For this review, take the finished solid that the model builds, in its own axes (mm). A direction names the side the tool comes from. Coordinates: 2 decimals unless noted, no trailing zeros. Loops run counter-clockwise (first coordinate to the right, second up) from the corner with the lowest first, then second, coordinate; pieces in that order, holes last. Notation, with made-up numbers: (24, -13.75) - (81, -13.75) arc R19 ccw to (81, 13.25) - close; hole circle Ø3 at (16.5, 10.5). An arc over 180 degrees is marked (long way). One line per item, written item: value. Start each with the question number.
1. The part is to be moulded in two halves that separate along Y. For faces 3 (the face through (-1.46, 7.41, -35.94)), 4 (the face through (-1.46, 69.41, -35.94)), 5 (the face through (0, 0, -36)), 6 (the face through (-50, 197, -20)), say which applies: released by +Y, released by -Y, zero draft, split by the parting line, or undercut.
2. Insertion check: pin 1 (17.5 mm diameter, centred on x = 0, y = 14, fed in from -Z); pin 2 (23.5 mm diameter, centred on x = 9.5, y = 253.5, fed in from +Z). Each pin has a flat end and moves straight along its axis. Give the tip position at first contact, or say it passes through.
3. Take a section at D-D, the plane y = 366. State the section outline as (x, z) points, and give its area (3 significant figures).
4. Take a section at A-A, the plane z = -16. State the section outline as (x, y) points.
5. For faces 1 (the face through (42, 197, -15)), 2 (the face through (3.63, 391.69, -35.94)), list the 3-axis set-ups (+Z, -Z, +X, -X, +Y, -Y) from which the entire face can be reached by the end or side of a thin tool; tool diameter is ignored.
6. To check wall thickness, follow line 1 (X direction, y = 181, z = -28.5); line 2 (Z direction, x = -21.5, y = 25); line 3 (X direction, y = 219, z = -2). State the ranges of each line that lie inside material, in increasing order. Write a range as from..to.
7. Take a section at B-B, the plane y = 138. State the section outline as (x, z) points, and give its area (3 significant figures).
8. Take a section at C-C, the plane x = 19.5. State the section outline as (y, z) points.
```python
from build123d import *

# Parameters (mm, degrees)
EXTRUIR_L_MINA1_DEPTH         = 400
REDONDEO1_R                   = 3
REDONDEO2_R                   = 3
TALADRO_DE_MARGEN_PARA_M121_D = 13.5


with BuildPart() as part:
    # Croquis1 → Extruir-Lámina1 (new body)
    with BuildSketch(Plane(origin=(0, 0, 0), x_dir=(1, 0, 0), z_dir=(0, 1, 0))):
        with BuildLine():
            Line((50, 0), (50, 37))
            ThreePointArc((50, 37), (49.121320344, 39.121320344), (47, 40))
            Line((47, 40), (-47, 40))
            ThreePointArc((-47, 40), (-49.121320344, 39.121320344), (-50, 37))
            Line((-50, 37), (-50, 0))
            Line((-50, 0), (-42, 0))
            Line((-42, 0), (-42, 32))
            Line((-42, 32), (42, 32))
            Line((42, 32), (42, 0))
            Line((42, 0), (50, 0))
        make_face()
    extrude(amount=EXTRUIR_L_MINA1_DEPTH)

    # Redondeo1
    redondeo1_edges = [part.edges().sort_by_distance(p)[0] for p in [
        (42, 200, -32),
        (-42, 200, -32),
    ]]
    fillet(redondeo1_edges, radius=REDONDEO1_R)

    # Redondeo2
    redondeo2_edges = [part.edges().sort_by_distance(p)[0] for p in [
        (-50, 0, -18.5),
        (-49.121320344, 0, -39.121320344),
        (0, 0, -40),
        (49.121320344, 0, -39.121320344),
        (50, 0, -18.5),
        (50, 400, -18.5),
        (-50, 200, 0),
        (50, 200, 0),
        (49.121320344, 400, -39.121320344),
        (0, 400, -40),
        (-49.121320344, 400, -39.121320344),
        (42, 0, -14.5),
        (-50, 400, -18.5),
        (42, 400, -14.5),
        (0, 0, -32),
        (0, 400, -32),
        (41.121320344, 0, -31.121320344),
        (41.121320344, 400, -31.121320344),
        (-41.121320344, 0, -31.121320344),
        (-41.121320344, 400, -31.121320344),
        (-42, 400, -14.5),
        (-42, 0, -14.5),
    ]]
    fillet(redondeo2_edges, radius=REDONDEO2_R)

    # Taladro de margen para M121 (through all)
    with Locations(Plane(origin=(0, 0, -40), x_dir=(-1, 0, 0), z_dir=(0, 0, -1))):
        with Locations((0, 386), (0, 324), (0, 262), (0, 200), (0, 138), (0, 76), (0, 14)):
            Hole(TALADRO_DE_MARGEN_PARA_M121_D / 2)


solid = part.part
```
Solutions:
1. face 3: undercut
1. face 4: undercut
1. face 5: released by -Y
1. face 6: zero draft
2. pin 1: z = -40
2. pin 2: z = -32
3. outline: (-50, -37) arc R3 ccw to (-47, -40) - (47, -40) arc R3 ccw to (50, -37) - (50, -3) arc R3 ccw to (47, 0) - (42, 0) - (42, -29) arc R3 cw to (39, -32) - (-39, -32) arc R3 cw to (-42, -29) - (-42, 0) - (-47, 0) arc R3 ccw to (-50, -3) - close
3. area: 1,310 mm2
4. outline: (-50, 3) arc R3 ccw to (-47, 0) - (-45, 0) arc R3 ccw to (-42, 3) - (-42, 397) arc R3 ccw to (-45, 400) - (-47, 400) arc R3 ccw to (-50, 397) - close; (42, 3) arc R3 ccw to (45, 0) - (47, 0) arc R3 ccw to (50, 3) - (50, 397) arc R3 ccw to (47, 400) - (45, 400) arc R3 ccw to (42, 397) - close
5. face 1: +Z, +Y, -Y
5. face 2: +Z, -Z
6. line 1: -50..-42, 42..50
6. line 2: -40..-32
6. line 3: -49.83..-42, 42..49.83
7. outline: (-50, -37) arc R3 ccw to (-47, -40) - (-6.75, -40) - (-6.75, -32) - (-39, -32) arc R3 cw to (-42, -29) - (-42, 0) - (-47, 0) arc R3 ccw to (-50, -3) - close; (6.75, -40) - (47, -40) arc R3 ccw to (50, -37) - (50, -3) arc R3 ccw to (47, 0) - (42, 0) - (42, -29) arc R3 cw to (39, -32) - (6.75, -32) - close
7. area: 1,200 mm2
8. outline: (0, -37) arc R3 ccw to (3, -40) - (397, -40) arc R3 ccw to (400, -37) - (400, -35) arc R3 ccw to (397, -32) - (3, -32) arc R3 ccw to (0, -35) - close
